The figure shows three views and two pictorial views of one solid part (mm, origin at its lowest corner). Answer the questions. A direction names the side the tool comes from. Round coordinates to 2 decimals unless told otherwise and drop trailing zeros. Order: outer loops, then holes, each group sorted by start corner. A loop starts at its lowest first (then second) coordinate and runs counter-clockwise, first axis right, second up.
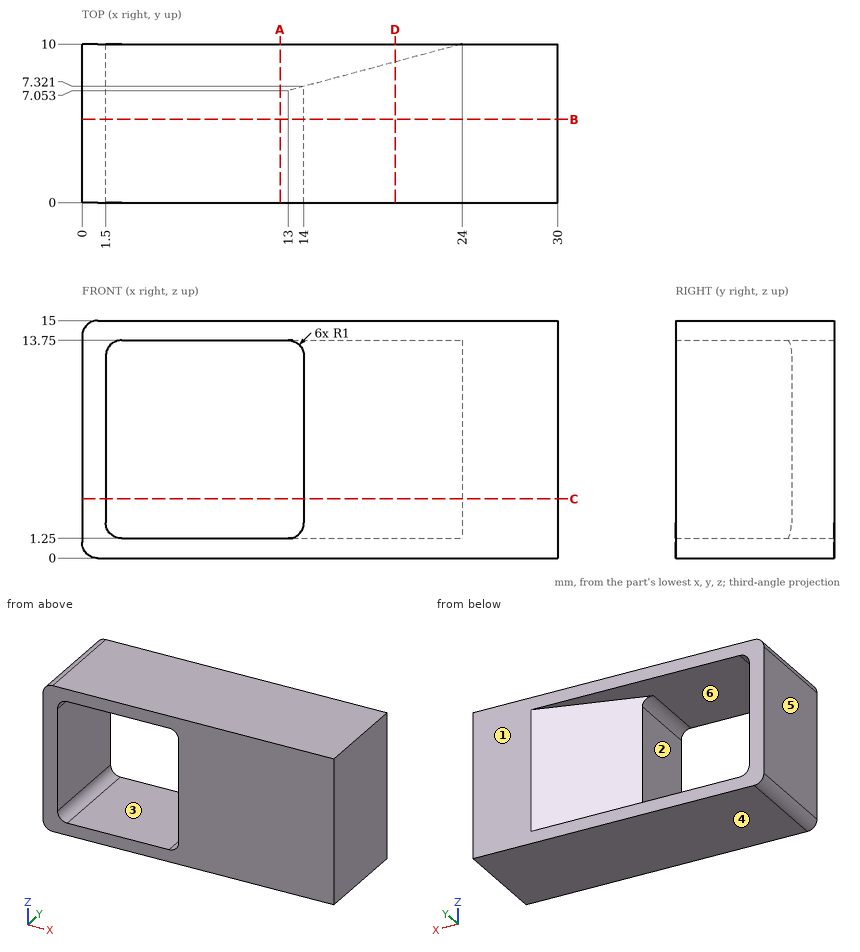
Item 1: Find the intervals of material crossed by line 1 along X through (y, z) = (2, 8.5); line 2 along Z through (x, y) = (5.5, 2.25); line 3 along X through (y, z) = (3, 13.25) (1 decimal), in increasing order.
Item 2: For a pull along X with two mould halves and no side action, classify the marked faces 4, 5 and 6 as released by +X, released by -X, zero draft, split by the parting line, or undercut.
Item 3: Find section B-B (y = 5.25). Write down the section's boundary in (x, z), plus the area to 3 significant figures.
Item 4: Find section C-C (z = 3.75). Write down the section's boundary in (x, y), plus the area to 3 significant figures.
Item 5: Given pin 1 (3 mm diameter, centred on x = 16, z = 6.5, fed in from +Y), flat-ended and moving along its own axis, determine where the tip first touches the part or whether it passes through.
Item 6: Find section D-D (x = 19.75). Write down the section's boundary in (y, z).
Item 7: Find section A-A (x = 12.5). Write down the section's boundary in (y, z).
Item 8: A tool of negligible diameter and unlimited length cuts with its end or side. For the marked faces 1, 2 and 3, from which of +Z, -Z, +X, -X, +Y, -Y can it reach the whole face along a straight path? Write none if from no direction.
Model answer:
1. line 1: x = 0 to 1.5, 14 to 30
1. line 2: z = 0 to 1.25, 13.75 to 15
1. line 3: x = 0 to 1.6, 13.9 to 30
2. face 4: zero draft
2. face 5: released by -X
2. face 6: undercut
3. outline: (0, 1) arc R1 ccw to (1, 0) - (30, 0) - (30, 15) - (1, 15) arc R1 ccw to (0, 14) - close; hole (1.5, 2.25) arc R1 ccw to (2.5, 1.25) - (13, 1.25) arc R1 ccw to (14, 2.25) - (14, 12.75) arc R1 ccw to (13, 13.75) - (2.5, 13.75) arc R1 ccw to (1.5, 12.75) - close
3. area: 294 mm2
4. outline: (0, 0) - (1.5, 0) - (1.5, 10) - (0, 10) - close; (14, 0) - (30, 0) - (30, 10) - (24, 10) - (14, 7.32) - close
4. area: 162 mm2
5. pin 1: stops at y = 8.26
6. outline: (0, 0) - (10, 0) - (10, 1.25) - (8.86, 1.25) - (8.86, 13.75) - (10, 13.75) - (10, 15) - (0, 15) - close
7. outline: (0, 0) - (10, 0) - (10, 1.25) - (0, 1.25) - close; (0, 13.75) - (10, 13.75) - (10, 15) - (0, 15) - close
8. face 1: +Z, -Z, +X, -X, +Y
8. face 2: +Y, -Y
8. face 3: +Y
